Geometry: final body of the model. Coordinates: model frame, mm. Coordinates: 2 decimals unless noted, no trailing zeros. Write each loop counter-clockwise with the first axis right and the second up, starting at its lowest first coordinate (ties: lowest second). Pieces come first, ordered by that corner, then holes. Notation, with made-up numbers: M -35,-10 L 18,-10 A8 ccw 18,-4 Z; hole C -19,-15 d6. An arc over 180 degrees is marked long. Write item = value, one per line. Start each with the question number.
Item 1: Section B-B on z = -169.5. Output: boundary loops of the cut face in (x, y).
Item 2: First-contact query: pin 1 Ø1 at (y, z) = (-6.5, -483.5) entering from +X; pin 2 Ø3 at (x, z) = (6.5, -65) entering from -Y; pin 3 Ø2 at (y, z) = (6, -426.5) entering from +X; pin 4 Ø8 at (x, y) = (0, 0) entering from -Z. Flat tips, straight axial feed; report the tip coordinate or a pass-through.
Item 3: Ray query, L1, parallel to Y at x = 0, z = -698.5; L2, parallel to Z at x = 5, y = 1; L3, parallel to Z at x = 8.5, y = -5. Return the intervals inside material, ascending. Write a range as [from, to].
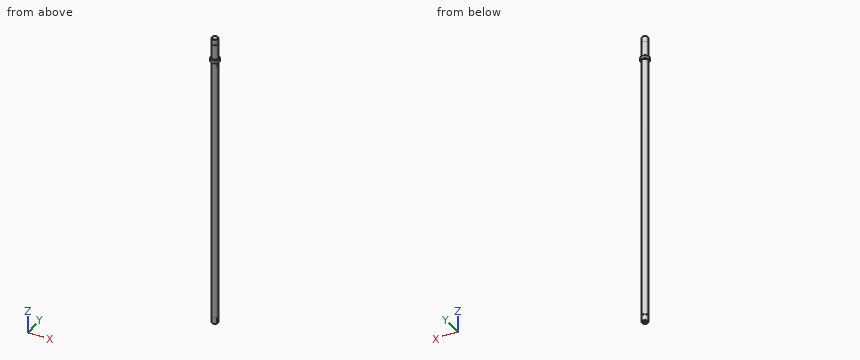
from build123d import *

# Parameters (mm, degrees)
CUT_EXTRUDE_1_DEPTH = 704.220626831
CHAMFER_1_SIZE      = 1
SKETCH_3_R          = 3
CUT_EXTRUDE_2_DEPTH = 15
CHAMFER_2_SIZE      = 0.5


with BuildPart() as part:
    # 草图1 → 旋转1 (revolve)
    with BuildSketch(Plane(origin=(0, 0, 0), x_dir=(0, 0, -1), z_dir=(1, 0, 0)), mode=Mode.PRIVATE) as revolve_1_sk:
        Polygon((0, 0), (0, 7), (14, 7), (14, 7.5), (49, 7.5), (49, 10), (57, 10), (57, 7.5), (687.5, 7.5), (687.5, 7), (703, 7), (703, 0), align=None)
    revolve(revolve_1_sk.sketch.rotate(Axis((0, 0, 0), (0, 0, 1)), 90), axis=Axis((0, 0, 0), (0, 0, 1)))

    # 草图2 → 切除-拉伸1 (cut, through all)
    with BuildSketch(Plane(origin=(4.5, 0, 0), x_dir=(0, 0, -1), z_dir=(1, 0, 0))):
        with BuildLine():
            Line((60, 2.5), (68, 2.5))
            ThreePointArc((68, 2.5), (70.5, 0), (68, -2.5))
            Line((68, -2.5), (60, -2.5))
            ThreePointArc((60, -2.5), (57.5, 0), (60, 2.5))
        make_face()
        with BuildLine():
            Line((690, 2.5), (700, 2.5))
            ThreePointArc((700, 2.5), (702.5, 0), (700, -2.5))
            Line((700, -2.5), (690, -2.5))
            ThreePointArc((690, -2.5), (687.5, 0), (690, 2.5))
        make_face()
    extrude(amount=CUT_EXTRUDE_1_DEPTH, mode=Mode.SUBTRACT)

    # 倒角1
    chamfer_1_edges = [part.edges().sort_by_distance(p)[0] for p in [
        (10, 0, -49),
    ]]
    chamfer(chamfer_1_edges, length=CHAMFER_1_SIZE)

    # 草图3 → 切除-拉伸2 (cut)
    with BuildSketch(Plane(origin=(0, 0, -703), x_dir=(-1, 0, 0), z_dir=(0, 0, -1))):
        Circle(SKETCH_3_R)
    extrude(amount=-CUT_EXTRUDE_2_DEPTH, mode=Mode.SUBTRACT)

    # 倒角2
    chamfer_2_edges = [part.edges().sort_by_distance(p)[0] for p in [
        (7, 0, 0),
        (3, 0, -703),
        (7, 0, -703),
    ]]
    chamfer(chamfer_2_edges, length=CHAMFER_2_SIZE - 0.0001)  # a hair under: the kernel refuses the full size


solid = part.part
Responses:
q1.outline = C 0,0 d15
q2.pin_1 = 4.5
q2.pin_2 = -5.59
q2.pin_3 = 5.59
q2.pin_4 = -703
q3.L1 = [-7, -3], [3, 7]
q3.L2 = [-703, -702.29], [-687.71, -70.29], [-57.71, 0]
q3.L3 = [-57, -49.86]
